Check sheet for the drawn part. Datum: minimum x, y, z corner. Units: mm. Coordinates: 2 decimals unless noted, no trailing zeros. Loops run counter-clockwise (first coordinate to the right, second up) from the corner with the lowest first, then second, coordinate; pieces in that order, holes last.
Q1. Sectioned sample at C-C (x = 30). Enter the section's corners in (y, z).
Q2. Sectioned sample at D-D (z = 3.2). Enter the section's corners in (x, y).
Q3. Sectioned sample at B-B (y = 18.5). Enter the section's corners in (x, z).
Q4. Material ranges on probe 1 along Y at (x, z) = (5.25, 2.85); probe 2 along Y at (x, z) = (4, 2.25); probe 3 along X at (y, z) = (56, 1.35), recorded low to high.
Q5. Go/stop test with a flat-tipped pin: P1, Ø4.5, axis at x = 54.75, y = 5.69, coming from the +Z side. Record where the tip stops, or that it passes through.
Q6. Sectioned sample at A-A (x = 54.75). Enter the section's corners in (y, z), then the cut area to 3 significant figures.
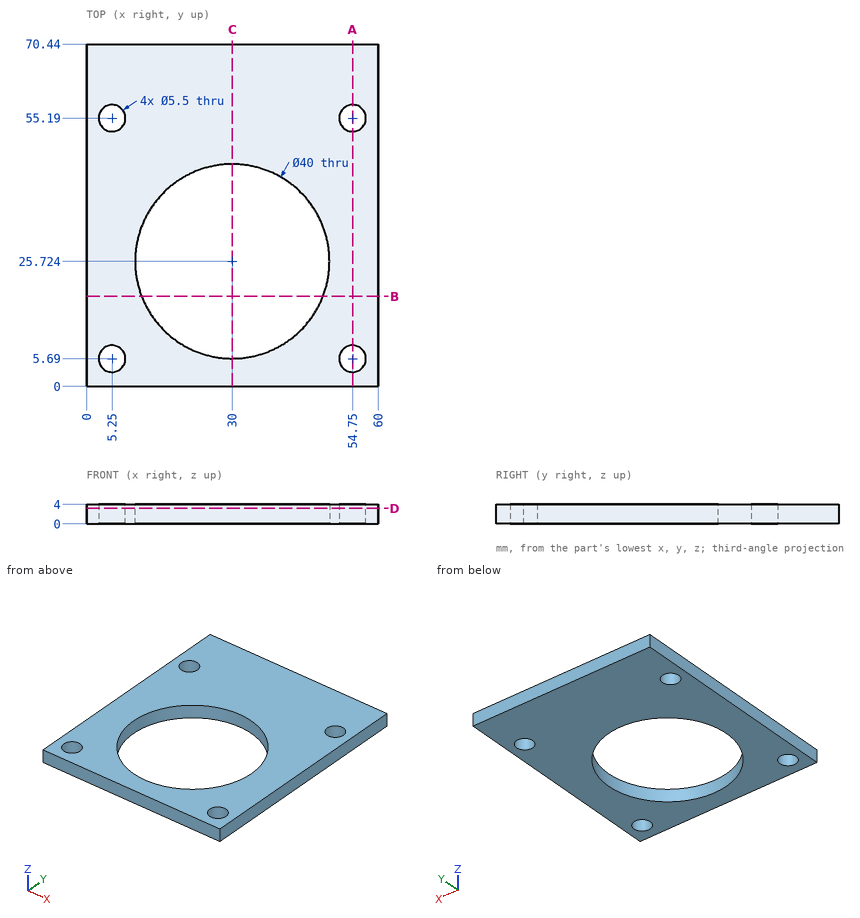
Geometry check:
1. outline: (0, 0) - (5.72, 0) - (5.72, 4) - (0, 4) - close; (45.72, 0) - (70.44, 0) - (70.44, 4) - (45.72, 4) - close
2. outline: (0, 0) - (60, 0) - (60, 70.44) - (0, 70.44) - close; hole circle Ø5.5 at (5.25, 5.69); hole circle Ø5.5 at (5.25, 55.19); hole circle Ø40 at (30, 25.72); hole circle Ø5.5 at (54.75, 5.69); hole circle Ø5.5 at (54.75, 55.19)
3. outline: (0, 0) - (11.35, 0) - (11.35, 4) - (0, 4) - close; (48.65, 0) - (60, 0) - (60, 4) - (48.65, 4) - close
4. probe 1: y = 0 to 2.94, 8.44 to 52.44, 57.94 to 70.44
4. probe 2: y = 0 to 3.24, 8.14 to 52.74, 57.64 to 70.44
4. probe 3: x = 0 to 2.62, 7.88 to 52.12, 57.38 to 60
5. P1: passes through
6. outline: (0, 0) - (2.94, 0) - (2.94, 4) - (0, 4) - close; (8.44, 0) - (52.44, 0) - (52.44, 4) - (8.44, 4) - close; (57.94, 0) - (70.44, 0) - (70.44, 4) - (57.94, 4) - close
6. area: 238 mm2
